Geometry check sheet. Reference: the model listing, model coordinates, mm. A direction names the side the tool comes from. Give positions to 0.01 mm unless a question says otherwise; leave off trailing zeros. Order: outer loops, then holes, each group sorted by start corner. A loop starts at its lowest first (then second) coordinate and runs counter-clockwise, first axis right, second up.
from build123d import *

# Parameters (mm, degrees)
SKETCH1_W           = 94.5
SKETCH1_H           = 90
SKETCH1_R           = 2
SKETCH1_R_2         = 2.5
SKETCH1_R_3         = 12.5
BOSS_EXTRUDE1_DEPTH = 10
SKETCH3_R           = 22.5
CUT_EXTRUDE2_DEPTH  = 3


with BuildPart() as part:
    # Sketch1 → Boss-Extrude1 (new body)
    with BuildSketch(Plane.XY):
        with Locations((47.25, 45)):
            Rectangle(SKETCH1_W, SKETCH1_H)
        with Locations((5, 80)):
            Circle(SKETCH1_R, mode=Mode.SUBTRACT)
        with Locations((5, 45)):
            Circle(SKETCH1_R, mode=Mode.SUBTRACT)
        with Locations(Location((5, 10, 0), (0, 0, 180))):
            Circle(SKETCH1_R, mode=Mode.SUBTRACT)
        with Locations((89.5, 10)):
            Circle(SKETCH1_R, mode=Mode.SUBTRACT)
        with Locations(Location((89.5, 45, 0), (0, 0, 180))):
            Circle(SKETCH1_R, mode=Mode.SUBTRACT)
        with Locations(Location((89.5, 80, 0), (0, 0, 180))):
            Circle(SKETCH1_R, mode=Mode.SUBTRACT)
        with Locations((24.75, 67.5)):
            Circle(SKETCH1_R_2, mode=Mode.SUBTRACT)
        with Locations((69.75, 67.5)):
            Circle(SKETCH1_R_2, mode=Mode.SUBTRACT)
        with Locations((69.75, 22.5)):
            Circle(SKETCH1_R_2, mode=Mode.SUBTRACT)
        with Locations((24.75, 22.5)):
            Circle(SKETCH1_R_2, mode=Mode.SUBTRACT)
        with Locations((47.25, 45)):
            Circle(SKETCH1_R_3, mode=Mode.SUBTRACT)
    extrude(amount=BOSS_EXTRUDE1_DEPTH)

    # Sketch3 → Cut-Extrude2 (cut)
    with BuildSketch(Plane.XY.offset(10)):
        with Locations((47.25, 45)):
            Circle(SKETCH3_R)
    extrude(amount=-CUT_EXTRUDE2_DEPTH, mode=Mode.SUBTRACT)


solid = part.part
Item 1: Gauge pin test, flat end, axial feed: pin 1 (8 mm diameter, centred on x = 69.75, y = 67.5, fed in from +Z). Record the tip position at first contact, or that the pin passes through.
Reported:
pin 1: stops at z = 10
Item 2: Draft check along Y on faces 1 (the flat face through (47, 0, 5)), 2 (the flat face through (36, 66, 10)), 3 (the cylindrical face through (5, 82, 5)). Enter one of: released by +Y, released by -Y, zero draft, split by the parting line, or undercut.
Reported:
face 1: released by -Y
face 2: zero draft
face 3: undercut
Item 3: Sectioned sample at A-A (y = 45). Enter the section's corners in (x, z), and give its area (3 significant figures).
Reported:
outline: (0, 0) - (3, 0) - (3, 10) - (0, 10) - close; (7, 0) - (34.75, 0) - (34.75, 7) - (24.75, 7) - (24.75, 10) - (7, 10) - close; (59.75, 0) - (87.5, 0) - (87.5, 10) - (69.75, 10) - (69.75, 7) - (59.75, 7) - close; (91.5, 0) - (94.5, 0) - (94.5, 10) - (91.5, 10) - close
area: 555 mm2
Item 4: Set-up check for faces 4 (the cylindrical face through (70.9, 65.28, 4.93)), 5 (the flat face through (57, 35, 7)): record each of +Z, -Z, +X, -X, +Y, -Y from which the full face is reachable in a straight line by a thin tool's end or side.
Reported:
face 4: +Z, -Z
face 5: +Z
Item 5: Sectioned sample at D-D (x = 89.5). Enter the section's corners in (y, z).
Reported:
outline: (0, 0) - (8, 0) - (8, 10) - (0, 10) - close; (12, 0) - (43, 0) - (43, 10) - (12, 10) - close; (47, 0) - (78, 0) - (78, 10) - (47, 10) - close; (82, 0) - (90, 0) - (90, 10) - (82, 10) - close
Item 6: Scan lines: L1, parallel to Y at x = 89.5, z = 6.75; L2, parallel to Y at x = 6.5, z = 2.75; L3, parallel to X at y = 11, z = 0.5. Record each from-to range of solid material in increasing order.
Reported:
L1: y = 0 to 8, 12 to 43, 47 to 78, 82 to 90
L2: y = 0 to 8.68, 11.32 to 43.68, 46.32 to 78.68, 81.32 to 90
L3: x = 0 to 3.27, 6.73 to 87.77, 91.23 to 94.5
Item 7: Sectioned sample at B-B (z = 2.5). Give the number of separate pieces and of enclosed holes in the cut face, and give its area (3 significant figures).
Reported:
separate pieces: 1
enclosed holes: 11
area: 7,860 mm2
Item 8: Sectioned sample at C-C (x = 47.25). Enter the section's corners in (y, z).
Reported:
outline: (0, 0) - (32.5, 0) - (32.5, 7) - (22.5, 7) - (22.5, 10) - (0, 10) - close; (57.5, 0) - (90, 0) - (90, 10) - (67.5, 10) - (67.5, 7) - (57.5, 7) - close
